```python
from build123d import *

# Parameters (mm, degrees)
SKETCH1_W                     = 19.05
SKETCH1_H                     = 19.05
SKETCH1_W_2                   = 15.875
SKETCH1_H_2                   = 15.875
BOSS_EXTRUDE1_DEPTH           = 104.775
SHELFBARMOUNTHOLE_REACH       = 108.918
SKETCH3_R                     = 2.4257
POWERSUPPLY_MOUNT_HOLES_REACH = 108.918
SKETCH4_R                     = 2.4257


with BuildPart() as part:
    # Sketch1 → Boss-Extrude1 (new, symmetric)
    with BuildSketch(Plane(origin=(0, 0, 0), x_dir=(0, -1, 0), z_dir=(1, 0, 0))):
        Rectangle(SKETCH1_W, SKETCH1_H)
        Rectangle(SKETCH1_W_2, SKETCH1_H_2, mode=Mode.SUBTRACT)
    extrude(amount=BOSS_EXTRUDE1_DEPTH, both=True)

    # Sketch3 → ShelfBarMountHole (cut, up to next)
    with BuildSketch(Plane.XZ.offset(9.525), mode=Mode.PRIVATE) as shelfbarmounthole_sk1:
        with Locations(Location((58.025000028, 0, 0), (0, 0, 270))):
            Circle(SKETCH3_R)
    shelfbarmounthole_tool1 = extrude(shelfbarmounthole_sk1.sketch, amount=-SHELFBARMOUNTHOLE_REACH, mode=Mode.PRIVATE) & part.part
    add(shelfbarmounthole_tool1.solids().sort_by_distance((58.025, -9.525, 0))[0], mode=Mode.SUBTRACT)

    # Sketch4 → PowerSupply Mount Holes (cut, up to next)
    with BuildSketch(Plane.XY.offset(-9.525), mode=Mode.PRIVATE) as powersupply_mount_holes_sk1:
        with Locations((-66.675, 0)):
            Circle(SKETCH4_R)
    powersupply_mount_holes_tool1 = extrude(powersupply_mount_holes_sk1.sketch, amount=POWERSUPPLY_MOUNT_HOLES_REACH, mode=Mode.PRIVATE) & part.part
    # Sketch4 → PowerSupply Mount Holes (cut, up to next)
    with BuildSketch(Plane.XY.offset(-9.525), mode=Mode.PRIVATE) as powersupply_mount_holes_sk2:
        with Locations((73.025, 0)):
            Circle(SKETCH4_R)
    powersupply_mount_holes_tool2 = extrude(powersupply_mount_holes_sk2.sketch, amount=POWERSUPPLY_MOUNT_HOLES_REACH, mode=Mode.PRIVATE) & part.part
    add(powersupply_mount_holes_tool1.solids().sort_by_distance((-66.675, 0, -9.525))[0], mode=Mode.SUBTRACT)
    add(powersupply_mount_holes_tool2.solids().sort_by_distance((73.025, 0, -9.525))[0], mode=Mode.SUBTRACT)


solid = part.part
```
Read the model definition and answer for the solid it produces. Units are mm, in the model's axes. A direction names the side the tool comes from. Round coordinates to 2 decimals unless told otherwise and drop trailing zeros. Write each loop counter-clockwise with the first axis right and the second up, starting at its lowest first coordinate (ties: lowest second). Pieces come first, ordered by that corner, then holes. Notation, with made-up numbers: (-12.5, -38) -> (34.5, -38) arc R29 ccw to (34.5, -1) -> close; hole circle Ø6 at (67.5, -3). An arc over 180 degrees is marked (long way). Answer in a Markdown table with one row per item. Add a question column.
1) Find section C-C, the plane x = -89.5. Determine the outline of the cut face in (y, z) (1 decimal), and give its area (3 significant figures).
2) Determine the mould class of faces 1 (the face through (104.775, 9, 0)), 2 (the face through (1, 0, -9.525)), 3 (the face through (-69.1, 0.1, -8.7)), 4 (the face through (60.43, -8.74, 0.32)) for opening direction X: pulls with the +X half, pulls with the -X half, needs draft (parallel to the pull), parting line crosses it, or undercut.
3) Find section B-B, the plane y = 0. Determine the outline of the cut face in (x, z) (1 decimal).
4) Consider line 1 (X direction, y = 0, z = -8.6) (3 decimals); line 2 (Z direction, x = 48, y = 6.25) (1 decimal); line 3 (X direction, y = -8.45, z = 0) (3 decimals). Determine where each line is inside the solid, lowest interval first.
5) Which of the six approach directions +Z, -Z, +X, -X, +Y, -Y give full straight-line access (tool end or side, diameter ignored) to faces 5 (the face through (1, 0, -7.938)), 6 (the face through (75.34, 0.73, -8.74)), 7 (the face through (1, 0, 9.525))?
6) Find section A-A, the plane z = 0. Determine the outline of the cut face in (x, y) (1 decimal).
7) Given P1, Ø3, axis at y = 0.5, z = 6, coming from the -X side, flat-ended and moving along its own axis, determine where the tip first touches the part or whether it passes through.
Findings below:
| question | item | result |
|---|---|---|
| 1 | outline | (-9.5, -9.5) -> (9.5, -9.5) -> (9.5, 9.5) -> (-9.5, 9.5) -> close; hole (-7.9, -7.9) -> (7.9, -7.9) -> (7.9, 7.9) -> (-7.9, 7.9) -> close |
| 1 | area | 111 mm² |
| 2 | face 1 | pulls with the +X half |
| 2 | face 2 | needs draft |
| 2 | face 3 | undercut |
| 2 | face 4 | undercut |
| 3 | outline | (-104.8, -9.5) -> (-69.1, -9.5) -> (-69.1, -7.9) -> (-104.8, -7.9) -> close; (-104.8, 7.9) -> (104.8, 7.9) -> (104.8, 9.5) -> (-104.8, 9.5) -> close; (-64.2, -9.5) -> (70.6, -9.5) -> (70.6, -7.9) -> (-64.2, -7.9) -> close; (75.5, -9.5) -> (104.8, -9.5) -> (104.8, -7.9) -> (75.5, -7.9) -> close |
| 4 | line 1 | -104.775 to -69.101, -64.249 to 70.599, 75.451 to 104.775 |
| 4 | line 2 | -9.5 to -7.9, 7.9 to 9.5 |
| 4 | line 3 | -104.775 to 55.599, 60.451 to 104.775 |
| 5 | face 5 | +X, -X |
| 5 | face 6 | -Z |
| 5 | face 7 | +Z, +X, -X, +Y, -Y |
| 6 | outline | (-104.8, -9.5) -> (55.6, -9.5) -> (55.6, -7.9) -> (-104.8, -7.9) -> close; (-104.8, 7.9) -> (104.8, 7.9) -> (104.8, 9.5) -> (-104.8, 9.5) -> close; (60.5, -9.5) -> (104.8, -9.5) -> (104.8, -7.9) -> (60.5, -7.9) -> close |
| 7 | P1 | through |
